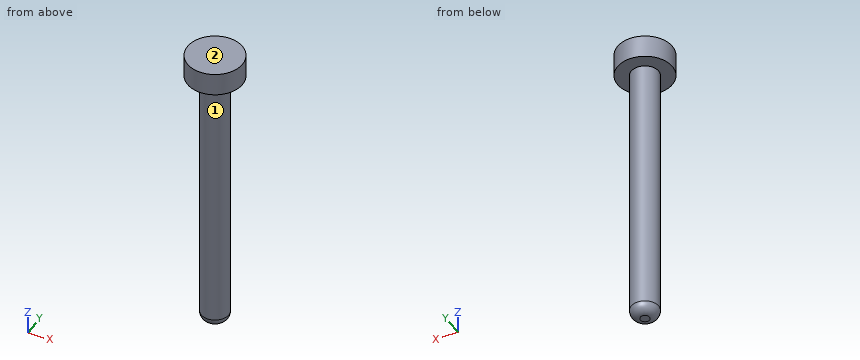
from build123d import *

# Parameters (mm, degrees)
SKETCH1_R           = 3
BOSS_EXTRUDE1_DEPTH = 65
SKETCH2_R           = 6
BOSS_EXTRUDE2_DEPTH = 5
FILLET1_R           = 2


with BuildPart() as part:
    # Sketch1 → Boss-Extrude1 (new body)
    with BuildSketch(Plane.XY):
        Circle(SKETCH1_R)
    extrude(amount=BOSS_EXTRUDE1_DEPTH)

    # Sketch2 → Boss-Extrude2 (add)
    with BuildSketch(Plane.XY.offset(65)):
        Circle(SKETCH2_R)
    extrude(amount=-BOSS_EXTRUDE2_DEPTH)

    # Fillet1
    fillet1_edges = [part.edges().sort_by_distance(p)[0] for p in [
        (-3, 0, 0),
    ]]
    fillet(fillet1_edges, radius=FILLET1_R)


solid = part.part
The listing builds one solid part. Answer for the finished solid, in the listing's coordinates (mm). Face numbers are marked on the shaded views. A direction names the side the tool comes from. Round coordinates to 2 decimals unless told otherwise and drop trailing zeros. Write each loop counter-clockwise with the first axis right and the second up, starting at its lowest first coordinate (ties: lowest second). Pieces come first, ordered by that corner, then holes. Notation, with made-up numbers: M 34.25,-0.5 L 74.25,-0.5 A18 cw 74.25,9.5 Z; hole C 78.25,58 d9. An arc over 180 degrees is marked long. Write each question's results on one line, items separated by ' | '. Start each with the question number.
(1) The part is cut by section B-B, the plane x = 5.25. Write down the section's boundary in (y, z).
(2) The part is cut by section A-A, the plane z = 25. Write down the section's boundary in (x, y).
(3) The part is cut by section C-C, the plane y = 4. Write down the section's boundary in (x, z), and give its area (3 significant figures).
(4) Each of these flat-tipped pins is pushed along its axis until it touches: P1, Ø4, axis at y = 0, z = 10.5, coming from the +X side; P2, Ø2, axis at x = -3, z = 57.5, coming from the -Y side; P3, Ø6, axis at x = 3.5, z = 13.5, coming from the +Y side. Where does it stop, or does it pass through?
(5) For the marked faces 1 and 2, determine the directions among +Z, -Z, +X, -X, +Y, -Y from which every point of the face is accessible in a straight line to the end or side of a thin tool.
(6) Find the intervals of material crossed by line 1 (Y direction, x = 0, z = 28.5); line 2 (Z direction, x = -5, y = -2.75); line 3 (X direction, y = 0.25, z = 11.5), in increasing order.
Worked answers:
1) outline: M -2.9,60 L 2.9,60 L 2.9,65 L -2.9,65 Z
2) outline: C 0,0 d6
3) outline: M -4.47,60 L 4.47,60 L 4.47,65 L -4.47,65 Z | area: 44.7 mm²
4) P1: stops at x = 3 | P2: stops at y = -2.24 | P3: stops at y = 2.96
5) face 1: -Z | face 2: +Z, +X, -X, +Y, -Y
6) line 1: y = -3 to 3 | line 2: z = 60 to 65 | line 3: x = -2.99 to 2.99
